Autodesk Inventor part; units mm, degrees
ref_plane "YZ Plane" through (0, 0, 0) normal (1, 0, 0) x (0, 1, 0)
ref_plane "XZ Plane" through (0, 0, 0) normal (0, 1, 0) x (-1, 0, 0)
ref_plane "XY Plane" through (0, 0, 0) normal (0, 0, 1) x (1, 0, 0)
sketch "Esquisse2" plane through (0, 0, 0) normal (0, 1, 0) x (-1, 0, 0)
  circle A0 centre (0, 0) radius 7.6
  dimension "d0" = 15.2
extrude "Extrusion1" add sketch "Esquisse2" along normal blind 15
sketch "Esquisse4" plane through (0, 15, 0) normal (0, 1, 0) x (1, 0, 0)
  circle A0 centre (0, 0) radius 7.6
  circle A1 centre (0, 0) radius 7.6
  arc A2 (-3.2, -6.8935) -> (0, -7.6) centre (0, 0) ccw
  line L0 (-0.0062, -0.0113) -> (-4.6214, -8.4012)
  line L1 (0, -6.3735) -> (0, 5.2233) construction
  line L2 (-3.2, -6.8935) -> (0, -7.6) construction
  line L3 (-3.2, -6.8935) -> (-3.0675, -6.2935)
  line L4 (0, -7.6) -> (0.1325, -7)
  arc A3 (0.1325, -7) -> (-3.0675, -6.2935) centre (-1.4675, -6.6467) ccw
  line L5 (-3.0675, -6.2935) -> (0.1325, -7) construction
  arc A4 (-6.419, -4.069) -> (-4.109, -6.3935) centre (0, 0) ccw
  line L6 (-4.109, -6.3935) -> (-6.419, -4.069) construction
  line L7 (-4.109, -6.3935) -> (-3.6731, -5.9603)
  line L8 (-6.419, -4.069) -> (-5.9831, -3.6359)
  arc A5 (-3.6731, -5.9603) -> (-5.9831, -3.6359) centre (-4.8281, -4.7981) ccw
  line L9 (-3.6731, -5.9603) -> (-5.9831, -3.6359) construction
  line L10 (-4.109, -6.3935) -> (-3.2, -6.8935) construction
  line L11 (0, 0) -> (-8.9658, -4.8594)
  arc A6 (-6.3677, 4.1487) -> (-7.5226, 1.0819) centre (0, 0) ccw
  line L12 (-7.5226, 1.0819) -> (-6.3677, 4.1487) construction
  line L13 (-7.5226, 1.0819) -> (-6.9476, 0.8653)
  line L14 (-6.3677, 4.1487) -> (-5.7927, 3.9322)
  arc A7 (-6.9476, 0.8653) -> (-5.7927, 3.9322) centre (-6.3701, 2.3988) ccw
  line L15 (-6.9476, 0.8653) -> (-5.7927, 3.9322) construction
  arc A8 (-7.5999, 0.0474) -> (-6.9133, -3.157) centre (0, 0) ccw
  line L16 (-7.5999, 0.0474) -> (-6.9133, -3.157) construction
  line L17 (-7.5999, 0.0474) -> (-6.999, 0.1761)
  line L18 (-6.9133, -3.157) -> (-6.3125, -3.0282)
  arc A9 (-6.3125, -3.0282) -> (-6.999, 0.1761) centre (-6.6558, -1.4261) ccw
  line L19 (-6.999, 0.1761) -> (-6.3125, -3.0282) construction
  line L20 (-7.5999, 0.0474) -> (-7.5226, 1.0819) construction
  line L21 (-6.9133, -3.157) -> (-6.419, -4.069) construction
  line L22 (0, 0) -> (-6.7758, 5.1057)
  arc A10 (7.3055, 2.0952) -> (5.7441, 4.9764) centre (0, 0) ccw
  line L23 (5.7441, 4.9764) -> (7.3055, 2.0952) construction
  line L24 (5.7441, 4.9764) -> (5.2039, 4.6837)
  line L25 (7.3055, 2.0952) -> (6.7653, 1.8025)
  arc A11 (5.2039, 4.6837) -> (6.7653, 1.8025) centre (5.9846, 3.2431) ccw
  line L26 (5.2039, 4.6837) -> (6.7653, 1.8025) construction
  arc A12 (5.0129, 5.7123) -> (2.1417, 7.292) centre (0, 0) ccw
  line L27 (5.0129, 5.7123) -> (2.1417, 7.292) construction
  line L28 (5.0129, 5.7123) -> (4.7167, 5.174)
  line L29 (2.1417, 7.292) -> (1.8455, 6.7536)
  arc A13 (1.8455, 6.7536) -> (4.7167, 5.174) centre (3.2811, 5.9638) ccw
  line L30 (4.7167, 5.174) -> (1.8455, 6.7536) construction
  line L31 (5.0129, 5.7123) -> (5.7441, 4.9764) construction
  line L32 (-3.1138, 6.9328) -> (-2.7472, 6.4398)
  arc A14 (-5.3768, 4.4842) -> (-2.7472, 6.4398) centre (-4.062, 5.462) ccw
  line L33 (-2.7472, 6.4398) -> (-5.3768, 4.4842) construction
  line L34 (-3.1138, 6.9328) -> (-5.7434, 4.9772) construction
  arc A15 (-3.1138, 6.9328) -> (-5.7434, 4.9772) centre (0, 0) ccw
  line L35 (-5.7434, 4.9772) -> (-5.3768, 4.4842)
  line L36 (-2.1407, 7.2923) -> (-3.1138, 6.9328) construction
  line L37 (-2.1407, 7.2923) -> (-2.0988, 6.6793)
  line L38 (-2.0988, 6.6793) -> (1.1706, 6.9027) construction
  line L39 (-2.1407, 7.2923) -> (1.1287, 7.5157) construction
  arc A16 (1.1287, 7.5157) -> (-2.1407, 7.2923) centre (0, 0) ccw
  arc A17 (-2.0988, 6.6793) -> (1.1706, 6.9027) centre (-0.4641, 6.791) ccw
  line L40 (1.1287, 7.5157) -> (1.1706, 6.9027)
  line L41 (1.1287, 7.5157) -> (2.1417, 7.292) construction
  line L42 (-6.3677, 4.1487) -> (-5.7434, 4.9772) construction
  line L43 (0, 0) -> (10.678, -14.3583) construction
  arc A18 (7.2785, -2.1871) -> (7.5228, 1.0808) centre (0, 0) ccw
  line L44 (7.5228, 1.0808) -> (7.2785, -2.1871) construction
  line L45 (7.5228, 1.0808) -> (6.91, 1.1266)
  line L46 (7.2785, -2.1871) -> (6.6658, -2.1413)
  arc A19 (6.91, 1.1266) -> (6.6658, -2.1413) centre (6.7879, -0.5073) ccw
  line L47 (6.91, 1.1266) -> (6.6658, -2.1413) construction
  line L48 (7.3055, 2.0952) -> (7.5228, 1.0808) construction
  line L49 (7.2785, -2.1871) -> (0, -7.6) construction
  line L50 (0, 0) -> (10.2791, -3.8716)
  line L51 (1.0339, -7.5293) -> (0.8211, -6.9529)
  arc A20 (3.8952, -5.8176) -> (0.8211, -6.9529) centre (2.3581, -6.3853) ccw
  arc A21 (1.0339, -7.5293) -> (4.1081, -6.394) centre (0, 0) ccw
  line L52 (4.1081, -6.394) -> (3.8952, -5.8176)
  line L53 (0.8211, -6.9529) -> (3.8952, -5.8176) construction
  line L54 (4.9405, -5.775) -> (4.4498, -5.4052)
  arc A22 (6.4221, -2.7881) -> (4.4498, -5.4052) centre (5.436, -4.0967) ccw
  line L55 (4.4498, -5.4052) -> (6.4221, -2.7881) construction
  line L56 (4.9405, -5.775) -> (6.9128, -3.1579) construction
  arc A23 (4.9405, -5.775) -> (6.9128, -3.1579) centre (0, 0) ccw
  line L57 (6.9128, -3.1579) -> (6.4221, -2.7881)
  line L58 (7.2785, -2.1871) -> (6.9128, -3.1579) construction
  point P0 (-7.5999, 0.0474)
  point P1 (-6.9133, -3.157)
  point P2 (-6.3677, 4.1487)
  point P3 (-7.5226, 1.0819)
  point P4 (-3.1138, 6.9328)
  point P5 (-5.7434, 4.9772)
  point P6 (1.1287, 7.5157)
  point P7 (-2.1407, 7.2923)
  point P8 (5.0129, 5.7123)
  point P9 (2.1417, 7.292)
  point P10 (7.3055, 2.0952)
  point P11 (5.7441, 4.9764)
  point P12 (-3.2, -6.8935)
  point P13 (0, -7.6)
  point P14 (-6.419, -4.069)
  point P15 (-4.109, -6.3935)
  point P16 (7.2785, -2.1871)
  point P17 (7.5228, 1.0808)
  point P18 (4.9405, -5.775)
  point P19 (4.9405, -5.775)
  point P20 (6.9128, -3.1579)
  point P21 (1.0339, -7.5293)
  point P22 (4.1081, -6.394)
  dimension "d14" = 3.2
  dimension "d28" = 0.6
  dimension "d30" = 0.5
extrude "Extrusion6" cut sketch "Esquisse4" against normal blind 15 contours A0 L46 A19 L45 | L25 A11 L24 A0 | A0 L54 A22 L57 | L28 A13 L29 A0 | A0 L51 A20 L52 | A0 L17 A9 L18 | L8 A5 L7 A0 | A0 L32 A14 L35 | L14 A7 L13 A0 | L40 A17 L37 A0 | A0 L3 A3 L4
sketch "Esquisse6" plane through (0, 15, 0) normal (0, 1, 0) x (1, 0, 0)
  circle A0 centre (0, 0) radius 9
  dimension "d19" = 18
extrude "Extrusion3" add sketch "Esquisse6" along normal blind 1.5
sketch "Esquisse7" plane through (0, 0, 0) normal (0, -1, 0) x (1, 0, 0)
  circle A0 centre (0, 0) radius 9
  dimension "d34" = 18
extrude "Extrusion4" add sketch "Esquisse7" along normal blind 1.5
sketch "Esquisse8" plane through (0, 16.5, 0) normal (0, 1, 0) x (1, 0, 0)
  circle A0 centre (0, 0) radius 4.5
  dimension "d24" = 9
extrude "Extrusion5" cut sketch "Esquisse8" against normal through all
properties part number "Pièce_moteur_courroie_test_4"
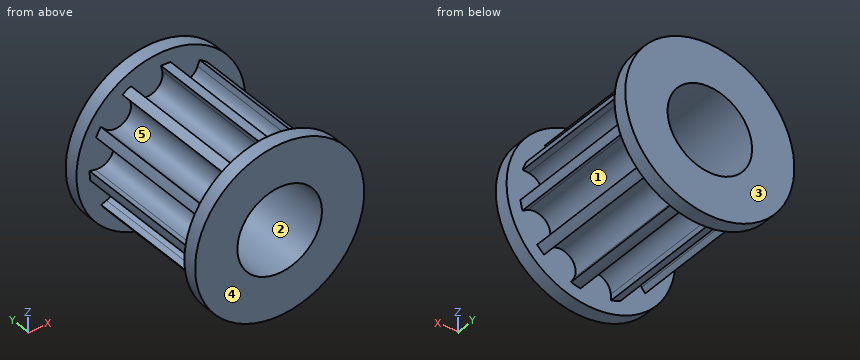
Build history of the part. All positions in model axes, mm. Face numbers are marked on the shaded views. A direction names the side the tool comes from. Round coordinates to 2 decimals unless told otherwise and drop trailing zeros. Write each loop counter-clockwise with the first axis right and the second up, starting at its lowest first coordinate (ties: lowest second). Pieces come first, ordered by that corner, then holes. Notation, with made-up numbers: (-35, -38.75) - (17, -38.75) arc R25 ccw to (17, -19.75) - close; hole circle Ø6 at (-12.5, 6.5). An arc over 180 degrees is marked (long way). Use CSV: the item, a comma, the result in double quotes.
(1) Pin check, flat tips, straight feed: P1, Ø6, axis at x = -2.5, z = -1, coming from the -Y side; P2, Ø3, axis at y = 12, z = 6.5, coming from the -X side; P3, Ø2, axis at x = -0.5, y = 13, coming from the -Z side. Stop position of each tip, or through.
Response:
P1,"y = -1.5"
P2,"x = -4.11"
P3,"z = -5.52"
(2) Band-saw the part on A-A (z = 1.5). Write the cut outline in (x, y), plus the area to 3 significant figures.
Response:
outline,"(-8.87, -1.5) - (-4.24, -1.5) - (-4.24, 16.5) - (-8.87, 16.5) - (-8.87, 15) - (-5.02, 15) - (-5.02, 0) - (-8.87, 0) - close; (4.24, -1.5) - (8.87, -1.5) - (8.87, 0) - (5.48, 0) - (5.48, 15) - (8.87, 15) - (8.87, 16.5) - (4.24, 16.5) - close"
area,"58.1 mm²"
(3) Wall check: line 1 (Y direction, x = 6.5, z = -4); line 2 (X direction, y = 4.5, z = 6.25); line 3 (X direction, y = 12, z = 3.5). Give the ranges that are in metal, low to high.
Response:
line 1,"-1.5 to 0, 15 to 16.5"
line 2,"-3.96 to -3.06, 0.12 to 0.73, 4.05 to 4.32"
line 3,"-6.75 to -5.83, -3.83 to -2.83, 2.83 to 3.91"
(4) 3-axis set-ups, long thin cutter, end or side, ignore diameter. For the marked faces 4 and 5: which of +Z, -Z, +X, -X, +Y, -Y reach the whole face in a straight line?
Response:
face 4,"+Z, -Z, +X, -X, -Y"
face 5,"none"
(5) Band-saw the part on C-C (z = -3.25). Write the cut outline in (x, y).
Response:
outline,"(-8.39, -1.5) - (-3.11, -1.5) - (-3.11, 16.5) - (-8.39, 16.5) - (-8.39, 15) - (-4.97, 15) - (-4.97, 0) - (-8.39, 0) - close; (3.11, -1.5) - (8.39, -1.5) - (8.39, 0) - (4.35, 0) - (4.35, 15) - (8.39, 15) - (8.39, 16.5) - (3.11, 16.5) - close"
(6) Band-saw the part on B-B (y = 15.25). Write the cut outline in (x, z), plus the area to 3 significant figures.
Response:
outline,"circle Ø18 at (0, 0); hole circle Ø9 at (0, 0)"
area,"191 mm²"
(7) Mould opens along Y. For the marked faces 1, 2 and 3 say: pulls with the +Y half, pulls with the -Y half, needs draft (parallel to the pull), parting line crosses it, or undercut.
Response:
face 1,"undercut"
face 2,"needs draft"
face 3,"pulls with the +Y half"
